Verification items for the finished model (mm, model axes). Round coordinates to 2 decimals unless told otherwise and drop trailing zeros. Write each loop counter-clockwise with the first axis right and the second up, starting at its lowest first coordinate (ties: lowest second). Pieces come first, ordered by that corner, then holes. Notation, with made-up numbers: (49, 81) -> (98, 81) arc R21 ccw to (98, 107) -> close; hole circle Ø11 at (4.5, 6). An arc over 180 degrees is marked (long way). Answer as a JSON object with one key per item and string values. Group by question number.
(1) Sectioned sample at C-C on x = -30.8. Record the cut outline in (y, z), and give its area (3 significant figures).
(2) Sectioned sample at B-B on z = 3.5. Record the cut outline in (x, y), and give its area (3 significant figures).
(3) Sectioned sample at A-A on y = 22. Record the cut outline in (x, z).
(4) Sectioned sample at D-D on x = 19.5. Record the cut outline in (y, z), and give its area (3 significant figures).
(5) Draft check along X on faces 1 (the face through (-52.673, 1.972, -14.43)), 2 (the face through (88, 18, 0)). Enter one of: released by +X, released by -X, zero draft, split by the parting line, or undercut.
(6) Gauge pin test, flat ends, axial feed: pin 1 Ø1.9 at (x, z) = (-73.8, -12.7) entering from +Y; pin 2 Ø5 at (x, z) = (-30.8, -12.7) entering from +Y; pin 3 Ø1.9 at (x, z) = (-80, 33.5) entering from +Y. Record the tip position at first contact, or that the pin passes through.
(7) Scan lines: L1, parallel to X at y = 7, z = -25.4; L2, parallel to Z at x = 30, y = 2; L3, parallel to X at y = 31, z = 28.5. Record each from-to range of solid material in increasing order. Write a range as from..to.
```python
from build123d import *

# Parameters (mm, degrees)
SKETCH1_W           = 170
SKETCH1_H           = 75
BOSS_EXTRUDE1_DEPTH = 40
SHELL1_T            = 3
FILLET1_R           = 5
SKETCH2_W           = 10
SKETCH2_H           = 17.5
SKETCH2_R           = 1.6
BOSS_EXTRUDE2_DEPTH = 10
FILLET2_R           = 4
SKETCH5_W           = 10
SKETCH5_H           = 8
SKETCH5_R           = 1.6
BOSS_EXTRUDE3_DEPTH = 27
FILLET3_R           = 4
MIRROR7_OUTLINE_W   = 10
MIRROR7_OUTLINE_H   = 8
MIRROR7_OUTLINE_R   = 1.6
MIRROR7_DEPTH       = 37
MIRROR7_2_OUTLINE_R = 1.6
MIRROR7_2_DEPTH     = 10
MIRROR9_OUTLINE_W   = 10
MIRROR9_OUTLINE_H   = 8
MIRROR9_OUTLINE_R   = 1.6
MIRROR9_DEPTH       = 37
MIRROR9_2_OUTLINE_R = 1.6
MIRROR9_2_DEPTH     = 10
FILLET5_R           = 4
SKETCH6_R           = 3.75
SKETCH6_R_2         = 1.6
BOSS_EXTRUDE4_DEPTH = 7
LPATTERN1_COUNT     = 4
LPATTERN1_PITCH     = 43


# Read off the part's stored shape, not the designer's step: Mirror7, Mirror9
# Some blends are built 0.0001 mm under size
with BuildPart() as part:
    # Sketch1 → Boss-Extrude1 (new body)
    with BuildSketch(Plane(origin=(0, 0, 0), x_dir=(1, 0, 0), z_dir=(0, 1, 0))):
        Rectangle(SKETCH1_W, SKETCH1_H)
    extrude(amount=BOSS_EXTRUDE1_DEPTH)

    # Shell1
    shell1_openings = [part.faces().sort_by_distance(p)[0] for p in [
        (0, 40, 0),
    ]]
    offset(amount=SHELL1_T, openings=shell1_openings, kind=Kind.INTERSECTION)

    # Fillet1
    # the kernel refuses this fillet: 5 mm, written as the material it takes off along each edge
    with BuildSketch(Plane(origin=(-88, 52.5, 40.5), x_dir=(1, 0, 0), z_dir=(0, -1, 0)), Plane(origin=(88, -15.5, 40.5), x_dir=(-1, 0, 0), z_dir=(0, 1, 0)), Plane(origin=(88, -15.5, -40.5), x_dir=(0, 0, 1), z_dir=(0, 1, 0)), Plane(origin=(-88, -15.5, -40.5), x_dir=(1, 0, 0), z_dir=(0, 1, 0))) as fillet1_piece_1:
        with BuildLine():
            CenterArc((FILLET1_R, -FILLET1_R), FILLET1_R, 90, 90)
            Line((0, -FILLET1_R), (0, 0))
            Line((0, 0), (FILLET1_R, 0))
        make_face()
    extrude(amount=68, mode=Mode.SUBTRACT)

    # Sketch2 → Boss-Extrude2 (add)
    with BuildSketch(Plane(origin=(0, 0, 0), x_dir=(1, 0, 0), z_dir=(0, 1, 0))):
        with Locations((-80, 28.75)):
            Rectangle(SKETCH2_W, SKETCH2_H)
        with Locations(Location((-80, 25.4, 0), (0, 0, 270))):
            Circle(SKETCH2_R, mode=Mode.SUBTRACT)
    extrude(amount=BOSS_EXTRUDE2_DEPTH)

    # Fillet2
    fillet2_edges = [part.edges().sort_by_distance(p)[0] for p in [
        (-85, 5, -20),
        (-75, 5, -20),
        (-75, 5, -37.5),
    ]]
    fillet(fillet2_edges, radius=FILLET2_R)

    # Sketch5 → Boss-Extrude3 (add)
    with BuildSketch(Plane(origin=(0, 10, 0), x_dir=(1, 0, 0), z_dir=(0, 1, 0))):
        with Locations((-80, 33.5)):
            Rectangle(SKETCH5_W, SKETCH5_H)
        with Locations(Location((-80, 33.5, 0), (0, 0, 270))):
            Circle(SKETCH5_R, mode=Mode.SUBTRACT)
    extrude(amount=BOSS_EXTRUDE3_DEPTH)

    # Fillet3
    fillet3_edges = [part.edges().sort_by_distance(p)[0] for p in [
        (-75, 23.5, -37.5),
    ]]
    fillet(fillet3_edges, radius=FILLET3_R)

    # Mirror7 outline → Mirror7 (add)
    with BuildSketch(Plane(origin=(0, 0, 0), x_dir=(1, 0, 0), z_dir=(0, 1, 0))):
        with Locations((-80, -33.5)):
            Rectangle(MIRROR7_OUTLINE_W, MIRROR7_OUTLINE_H)
        with Locations((-80, -33.5)):
            Circle(MIRROR7_OUTLINE_R, mode=Mode.SUBTRACT)
    extrude(amount=MIRROR7_DEPTH)

    # Mirror7 2 outline → Mirror7 2 (add)
    # profile 1 of 2: a face of its own
    with BuildSketch(Plane(origin=(0, 0, 0), x_dir=(1, 0, 0), z_dir=(0, 1, 0))):
        with BuildLine():
            Line((-85, -29.5), (-75, -29.5))
            Line((-75, -29.5), (-75, -24))
            ThreePointArc((-75, -24), (-76.171572875, -21.171572875), (-79, -20))
            Line((-79, -20), (-81, -20))
            ThreePointArc((-81, -20), (-83.828427125, -18.828427125), (-85, -16))
            Line((-85, -16), (-85, -29.5))
        make_face()
        with Locations((-80, -25.4)):
            Circle(MIRROR7_2_OUTLINE_R, mode=Mode.SUBTRACT)
    # profile 2 of 2: a face of its own
    with BuildSketch(Plane(origin=(0, 0, 0), x_dir=(1, 0, 0), z_dir=(0, 1, 0))):
        with Locations((-80, -33.5)):
            Circle(MIRROR7_2_OUTLINE_R)
    extrude(amount=MIRROR7_2_DEPTH)

    # Mirror9 outline → Mirror9 (add)
    # profile 1 of 2: a face of its own
    with BuildSketch(Plane(origin=(0, 0, 0), x_dir=(1, 0, 0), z_dir=(0, 1, 0))):
        with Locations((80, 33.5)):
            Rectangle(MIRROR9_OUTLINE_W, MIRROR9_OUTLINE_H)
        with Locations((80, 33.5)):
            Circle(MIRROR9_OUTLINE_R, mode=Mode.SUBTRACT)
    # profile 2 of 2: a face of its own
    with BuildSketch(Plane(origin=(0, 0, 0), x_dir=(1, 0, 0), z_dir=(0, 1, 0))):
        with Locations((80, -33.5)):
            Rectangle(MIRROR9_OUTLINE_W, MIRROR9_OUTLINE_H)
        with Locations((80, -33.5)):
            Circle(MIRROR9_OUTLINE_R, mode=Mode.SUBTRACT)
    extrude(amount=MIRROR9_DEPTH)

    # Mirror9 2 outline → Mirror9 2 (add)
    # profile 1 of 5: a face of its own
    with BuildSketch(Plane(origin=(0, 0, 0), x_dir=(1, 0, 0), z_dir=(0, 1, 0))):
        with BuildLine():
            ThreePointArc((75, 24), (76.171572875, 21.171572875), (79, 20))
            Line((79, 20), (85, 20))
            Line((85, 20), (85, 29.5))
            Line((85, 29.5), (75, 29.5))
            Line((75, 29.5), (75, 24))
        make_face()
        with Locations((80, 25.4)):
            Circle(MIRROR9_2_OUTLINE_R, mode=Mode.SUBTRACT)
    # profile 2 of 5: a face of its own
    with BuildSketch(Plane(origin=(0, 0, 0), x_dir=(1, 0, 0), z_dir=(0, 1, 0))):
        with BuildLine():
            Line((85, -29.5), (85, -20))
            Line((85, -20), (79, -20))
            ThreePointArc((79, -20), (76.171572875, -21.171572875), (75, -24))
            Line((75, -24), (75, -29.5))
            Line((75, -29.5), (85, -29.5))
        make_face()
        with Locations((80, -25.4)):
            Circle(MIRROR9_2_OUTLINE_R, mode=Mode.SUBTRACT)
    # profile 3 of 5: a face of its own
    with BuildSketch(Plane(origin=(0, 0, 0), x_dir=(1, 0, 0), z_dir=(0, 1, 0))):
        with BuildLine():
            ThreePointArc((71, 37.5), (73.828427125, 36.328427125), (75, 33.5))
            Line((75, 33.5), (75, 37.5))
            Line((75, 37.5), (71, 37.5))
        make_face()
    # profile 4 of 5: a face of its own
    with BuildSketch(Plane(origin=(0, 0, 0), x_dir=(1, 0, 0), z_dir=(0, 1, 0))):
        with Locations((80, -33.5)):
            Circle(MIRROR9_2_OUTLINE_R)
    # profile 5 of 5: a face of its own
    with BuildSketch(Plane(origin=(0, 0, 0), x_dir=(1, 0, 0), z_dir=(0, 1, 0))):
        with Locations((80, 33.5)):
            Circle(MIRROR9_2_OUTLINE_R)
    extrude(amount=MIRROR9_2_DEPTH)

    # Fillet5
    fillet5_edges = [part.edges().sort_by_distance(p)[0] for p in [
        (75, 18.5, 37.5),
        (85, 5, 20),
        (85, 5, -20),
        (75, 23.5, -37.5),
        (-75, 18.5, 37.5),
    ]]
    fillet(fillet5_edges, radius=FILLET5_R - 0.0001)  # a hair under: the kernel refuses the full size

    # Sketch6 → Boss-Extrude4 (add)
    # profile 1 of 4: a face of its own
    with BuildSketch(Plane(origin=(0, -3, 0), x_dir=(1, 0, 0), z_dir=(0, 1, 0))):
        with Locations(Location((-56, 12.7, 0), (0, 0, 90))):
            Circle(SKETCH6_R)
        with Locations(Location((-56, 12.7, 0), (0, 0, 90))):
            Circle(SKETCH6_R_2, mode=Mode.SUBTRACT)
    # profile 2 of 4: a face of its own
    with BuildSketch(Plane(origin=(0, -3, 0), x_dir=(1, 0, 0), z_dir=(0, 1, 0))):
        with Locations(Location((-56, -12.7, 0), (0, 0, 90))):
            Circle(SKETCH6_R)
        with Locations(Location((-56, -12.7, 0), (0, 0, 90))):
            Circle(SKETCH6_R_2, mode=Mode.SUBTRACT)
    # profile 3 of 4: a face of its own
    with BuildSketch(Plane(origin=(0, -3, 0), x_dir=(1, 0, 0), z_dir=(0, 1, 0))):
        with Locations(Location((-73.8, 12.7, 0), (0, 0, 90))):
            Circle(SKETCH6_R)
        with Locations(Location((-73.8, 12.7, 0), (0, 0, 90))):
            Circle(SKETCH6_R_2, mode=Mode.SUBTRACT)
    # profile 4 of 4: a face of its own
    with BuildSketch(Plane(origin=(0, -3, 0), x_dir=(1, 0, 0), z_dir=(0, 1, 0))):
        with Locations(Location((-73.8, -12.7, 0), (0, 0, 90))):
            Circle(SKETCH6_R)
        with Locations(Location((-73.8, -12.7, 0), (0, 0, 90))):
            Circle(SKETCH6_R_2, mode=Mode.SUBTRACT)
    boss_extrude4 = extrude(amount=BOSS_EXTRUDE4_DEPTH)

    # LPattern1: Boss-Extrude4 ×4
    with Locations(*[(i * LPATTERN1_PITCH, 0, 0) for i in range(1, LPATTERN1_COUNT)]):
        add(boss_extrude4)


solid = part.part
```
Computed values:
{
 "1": {"outline": "(-3, -40.5) -> (40, -40.5) -> (40, -37.5) -> (0, -37.5) -> (0, -16.45) -> (4, -16.45) -> (4, -14.3) -> (0, -14.3) -> (0, -11.1) -> (4, -11.1) -> (4, -8.95) -> (0, -8.95) -> (0, 8.95) -> (4, 8.95) -> (4, 11.1) -> (0, 11.1) -> (0, 14.3) -> (4, 14.3) -> (4, 16.45) -> (0, 16.45) -> (0, 37.5) -> (40, 37.5) -> (40, 40.5) -> (-3, 40.5) -> close", "area": "517 mm2"},
 "2": {"outline": "(-88, -3) -> (88, -3) -> (88, 40) -> (85, 40) -> (85, 0) -> (-85, 0) -> (-85, 40) -> (-88, 40) -> close", "area": "768 mm2"},
 "3": {"outline": "(-88, -35.5) arc R5 ccw to (-83, -40.5) -> (83, -40.5) arc R5 ccw to (88, -35.5) -> (88, 35.5) arc R5 ccw to (83, 40.5) -> (-83, 40.5) arc R5 ccw to (-88, 35.5) -> close; hole (-85, -29.5) -> (-75, -29.5) -> (-75, -33.5) arc R4 ccw to (-71, -37.5) -> (71, -37.5) arc R4 ccw to (75, -33.5) -> (75, -29.5) -> (85, -29.5) -> (85, 29.5) -> (75, 29.5) -> (75, 33.5) arc R4 ccw to (71, 37.5) -> (-71, 37.5) arc R4 ccw to (-75, 33.5) -> (-75, 29.5) -> (-85, 29.5) -> close; hole circle Ø3.2 at (-80, -33.5); hole circle Ø3.2 at (-80, 33.5); hole circle Ø3.2 at (80, -33.5); hole circle Ø3.2 at (80, 33.5)"},
 "4": {"outline": "(-3, -40.5) -> (40, -40.5) -> (40, -37.5) -> (0, -37.5) -> (0, 37.5) -> (40, 37.5) -> (40, 40.5) -> (-3, 40.5) -> close", "area": "483 mm2"},
 "5": {"face 1": "undercut", "face 2": "released by +X"},
 "6": {"pin 1": "y = 0", "pin 2": "y = 4", "pin 3": "y = 10"},
 "7": {"L1": "-88..-81.6, -78.4..-75, 75..78.4, 81.6..88", "L2": "-40.5..-37.5, -16.45..-14.3, -11.1..-8.95, 8.95..11.1, 14.3..16.45, 37.5..40.5", "L3": "-88..-85, 85..88"}
}
